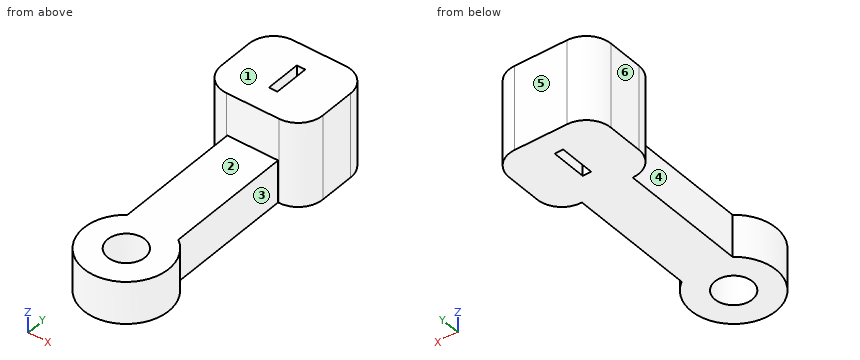
```python
from build123d import *

# Parameters (mm, degrees)
PAD_DEPTH       = 5
SKETCH001_W     = 12
SKETCH001_H     = 10
PAD001_DEPTH    = 5
SKETCH002_W     = 1
SKETCH002_H     = 4.2
POCKET_DEPTH    = 10
FILLET_R        = 2.9
FILLET001_R     = 2.9
FILLET002_R     = 2.9
FILLET003_R     = 2.9
SKETCH003_R     = 2.2
POCKET001_DEPTH = 5


with BuildPart() as part:
    # Sketch → Pad (new body)
    with BuildSketch(Plane.XY):
        with BuildLine():
            ThreePointArc((-3, 4), (0, -5), (3, 4))
            Line((3, 4), (3, 19))
            Line((6, 19), (3, 19))
            Line((6, 29), (6, 19))
            Line((-6, 29), (6, 29))
            Line((-6, 19), (-6, 29))
            Line((-3, 19), (-6, 19))
            Line((-3, 4), (-3, 19))
        make_face()
    extrude(amount=PAD_DEPTH)

    # Sketch001 (on Face10 of Pad) → Pad001 (join)
    with BuildSketch(Plane.XY.offset(5)):
        with Locations((0, 24)):
            Rectangle(SKETCH001_W, SKETCH001_H)
    extrude(amount=PAD001_DEPTH)

    # Sketch002 (on Face15 of Pad001) → Pocket (cut)
    with BuildSketch(Plane.XY.offset(10)):
        with Locations((0, 24.173883)):
            Rectangle(SKETCH002_W, SKETCH002_H)
    extrude(amount=-POCKET_DEPTH, mode=Mode.SUBTRACT)

    # Fillet
    fillet_edges = [part.edges().sort_by_distance(p)[0] for p in [
        (6, 19, 7.5),
    ]]
    fillet(fillet_edges, radius=FILLET_R)

    # Fillet001
    fillet001_edges = [part.edges().sort_by_distance(p)[0] for p in [
        (-6, 19, 7.5),
    ]]
    fillet(fillet001_edges, radius=FILLET001_R)

    # Fillet002
    fillet002_edges = [part.edges().sort_by_distance(p)[0] for p in [
        (6, 29, 7.5),
    ]]
    fillet(fillet002_edges, radius=FILLET002_R)

    # Fillet003
    fillet003_edges = [part.edges().sort_by_distance(p)[0] for p in [
        (-6, 29, 7.5),
    ]]
    fillet(fillet003_edges, radius=FILLET003_R)

    # Sketch003 (on Face26 of Fillet003) → Pocket001 (cut)
    with BuildSketch(Plane.XY.offset(5)):
        Circle(SKETCH003_R)
    extrude(amount=-POCKET001_DEPTH, mode=Mode.SUBTRACT)


solid = part.part
```
Geometry: final body of the model. Coordinates: model frame, mm. Face numbers are marked on the shaded views. A direction names the side the tool comes from. Coordinates: 2 decimals unless noted, no trailing zeros. Loops run counter-clockwise (first coordinate to the right, second up) from the corner with the lowest first, then second, coordinate; pieces in that order, holes last. Notation, with made-up numbers: (72.5, 68) -> (92.5, 68) arc R14 cw to (92.5, 86) -> close; hole circle Ø7 at (-17.5, 71.5). An arc over 180 degrees is marked (long way). Use a Markdown table: item, result. Add a question column.
(1) Section query D-D, the plane z = 9.25. Return loops of the section in (x, y).
(2) Mould query, pull axis Y, two halves, no side actions, for the marked faces 4, 5 and 6. Classes: pulls with the +Y half, pulls with the -Y half, needs draft (parallel to the pull), parting line crosses it, or undercut.
(3) Section query A-A, the plane x = 0. Return loops of the section in (y, z), plus the area to 3 significant figures.
(4) Access query for the marked faces 1, 2 and 3. Directions: +Z, -Z, +X, -X, +Y, -Y. A direction counts if a zero-diameter tool reaches every point of the face in a straight line with its end or side. Return the directions, or none.
(5) Pin query (flat end, axial travel): pin 1 Ø5.5 at (y, z) = (9.5, 3.5) entering from -X; pin 2 Ø4 at (x, y) = (0, 0) entering from +Z; pin 3 Ø1.5 at (x, y) = (-2.5, 15.5) entering from +Z; pin 4 Ø1 at (x, z) = (-4.5, 3) entering from -Y. Return the tip coordinate at first contact, or that it passes through.
(6) Line query: line 1 along Y through (x, z) = (0, 1.95); line 2 along X through (y, z) = (26, 8.5); line 3 along Y through (x, z) = (2.75, 9). Output: solid intervals per line, ascending.
(7) Section query C-C, the plane y = 0. Return loops of the section in (x, z).
(8) Section query B-B, the plane z = 2.5. Return loops of the section in (x, y).
Answer:
| question | item | result |
|---|---|---|
| 1 | outline | (-6, 21.9) arc R2.9 ccw to (-3.1, 19) -> (3.1, 19) arc R2.9 ccw to (6, 21.9) -> (6, 26.1) arc R2.9 ccw to (3.1, 29) -> (-3.1, 29) arc R2.9 ccw to (-6, 26.1) -> close; hole (-0.5, 22.07) -> (0.5, 22.07) -> (0.5, 26.27) -> (-0.5, 26.27) -> close |
| 2 | face 4 | undercut |
| 2 | face 5 | pulls with the +Y half |
| 2 | face 6 | needs draft |
| 3 | outline | (-5, 0) -> (-2.2, 0) -> (-2.2, 5) -> (-5, 5) -> close; (2.2, 0) -> (22.07, 0) -> (22.07, 10) -> (19, 10) -> (19, 5) -> (2.2, 5) -> close; (26.27, 0) -> (29, 0) -> (29, 10) -> (26.27, 10) -> close |
| 3 | area | 156 mm^2 |
| 4 | face 1 | +Z, +X, -X, +Y, -Y |
| 4 | face 2 | +Z, +X, -X, -Y |
| 4 | face 3 | +Z, -Z, +X |
| 5 | pin 1 | stops at x = -3 |
| 5 | pin 2 | passes through |
| 5 | pin 3 | stops at z = 5 |
| 5 | pin 4 | stops at y = -3 |
| 6 | line 1 | y = -5 to -2.2, 2.2 to 22.07, 26.27 to 29 |
| 6 | line 2 | x = -6 to -0.5, 0.5 to 6 |
| 6 | line 3 | y = 19 to 29 |
| 7 | outline | (-5, 0) -> (-2.2, 0) -> (-2.2, 5) -> (-5, 5) -> close; (2.2, 0) -> (5, 0) -> (5, 5) -> (2.2, 5) -> close |
| 8 | outline | (-6, 21.9) arc R2.9 ccw to (-3.1, 19) -> (-3, 19) -> (-3, 4) arc R5 ccw (long way) to (3, 4) -> (3, 19) -> (3.1, 19) arc R2.9 ccw to (6, 21.9) -> (6, 26.1) arc R2.9 ccw to (3.1, 29) -> (-3.1, 29) arc R2.9 ccw to (-6, 26.1) -> close; hole circle Ø4.4 at (0, 0); hole (-0.5, 22.07) -> (0.5, 22.07) -> (0.5, 26.27) -> (-0.5, 26.27) -> close |
